CAD build for the part. Positions are in the model's coordinates, mm. Face numbers are marked on the shaded views. A direction names the side the tool comes from. Round coordinates to 2 decimals unless told otherwise and drop trailing zeros. Order: outer loops, then holes, each group sorted by start corner. A loop starts at its lowest first (then second) coordinate and runs counter-clockwise, first axis right, second up. Notation, with made-up numbers: M 43.25,16 L 65.25,16 A27 cw 65.25,42 Z; hole C 65.5,76 d4. An arc over 180 degrees is marked long. Answer as a JSON object with one key per item and string values.
```python
from build123d import *

# Parameters (mm, degrees)
CUT_EXTRUDE1_DEPTH                = 145.941445074
CIRPATTERN1_COUNT                 = 6
CUT_EXTRUDE2_DEPTH                = 145.941445074
F_1_4_20_TAPPED_HOLE1_D           = 5.1054
F_1_4_20_TAPPED_HOLE1_DEPTH       = 12.7
F_1_4_20_TAPPED_HOLE1_CSINK_D     = 7.62
F_1_4_20_TAPPED_HOLE1_CSINK_ANGLE = 90
F_1_4_20_TAPPED_HOLE1_TIP         = 1.533816902


with BuildPart() as part:
    # Sketch1 → Revolve1 (revolve)
    with BuildSketch(Plane.XY, mode=Mode.PRIVATE) as revolve1_sk:
        Polygon((-6.35, 0), (6.35, 0), (6.35, 76.2), (7.62, 88.9), (12.7, 88.9), (12.7, 101.6), (-12.7, 101.6), (-12.7, 88.9), (-7.62, 88.9), (-6.35, 76.2), align=None)
    revolve(revolve1_sk.sketch.rotate(Axis((-21.230059302, 0, 0), (1, 0, 0)), 90), axis=Axis((-21.230059302, 0, 0), (1, 0, 0)))

    # Sketch2 → Cut-Extrude1 (cut, through all)
    with BuildSketch(Plane(origin=(6.35, 0, 0), x_dir=(0, 0, -1), z_dir=(1, 0, 0))):
        with BuildLine():
            Line((5.499261314, 34.925), (19.900738686, 59.869090512))
            ThreePointArc((19.900738686, 59.869090512), (19.900738686, 66.219090512), (14.401477372, 69.394090512))
            Line((14.401477372, 69.394090512), (-14.401477372, 69.394090512))
            ThreePointArc((-14.401477372, 69.394090512), (-19.900738686, 66.219090512), (-19.900738686, 59.869090512))
            Line((-19.900738686, 59.869090512), (-5.499261314, 34.925))
            ThreePointArc((-5.499261314, 34.925), (0, 31.75), (5.499261314, 34.925))
        make_face()
    cut_extrude1 = extrude(amount=-CUT_EXTRUDE1_DEPTH, mode=Mode.SUBTRACT)

    # CirPattern1: Cut-Extrude1 ×6 about axis
    cirpattern1_axis = Axis((0, 0, 0), (1, 0, 0))
    for i in range(1, CIRPATTERN1_COUNT):
        add(cut_extrude1.rotate(cirpattern1_axis, i * 360 / CIRPATTERN1_COUNT), mode=Mode.SUBTRACT)

    # Sketch3 → Cut-Extrude2 (cut, through all)
    with BuildSketch(Plane(origin=(6.35, 0, 0), x_dir=(0, 0, -1), z_dir=(1, 0, 0))):
        with BuildLine():
            Line((-6.35, 10.998522628), (-6.35, -10.998522628))
            ThreePointArc((-6.35, -10.998522628), (0, -12.7), (6.35, -10.998522628))
            Line((6.35, -10.998522628), (6.35, 10.998522628))
            ThreePointArc((6.35, 10.998522628), (0, 12.7), (-6.35, 10.998522628))
        make_face()
    extrude(amount=-CUT_EXTRUDE2_DEPTH, mode=Mode.SUBTRACT)

    # 1/4-20 Tapped Hole1
    with Locations(Plane(origin=(12.7, 0, 0), x_dir=(0, 0, -1), z_dir=(1, 0, 0))):
        with Locations((0, 95.25)):
            CounterSinkHole(F_1_4_20_TAPPED_HOLE1_D / 2, F_1_4_20_TAPPED_HOLE1_CSINK_D / 2, depth=F_1_4_20_TAPPED_HOLE1_DEPTH, counter_sink_angle=F_1_4_20_TAPPED_HOLE1_CSINK_ANGLE)
            with Locations((0, 0, -(F_1_4_20_TAPPED_HOLE1_DEPTH + F_1_4_20_TAPPED_HOLE1_TIP / 2))):  # 118° drill point
                Cone(0, F_1_4_20_TAPPED_HOLE1_D / 2, F_1_4_20_TAPPED_HOLE1_TIP, mode=Mode.SUBTRACT)


solid = part.part
```
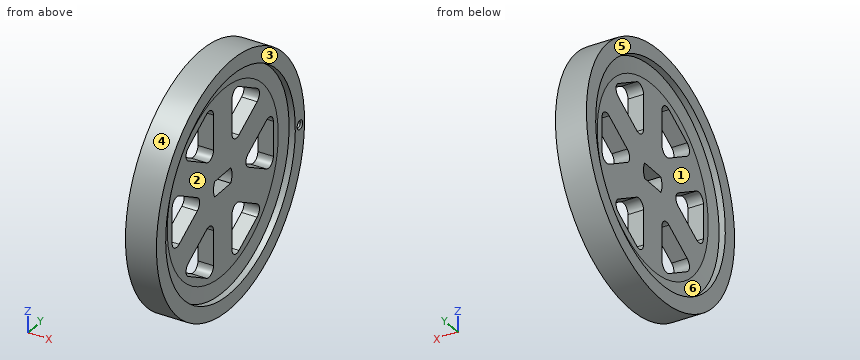
Item 1: 3-axis set-ups, long thin cutter, end or side, ignore diameter. For the marked faces 1, 2 and 3: which of +Z, -Z, +X, -X, +Y, -Y reach the whole face in a straight line?
Worked answers:
{"face 1": "-X", "face 2": "+X", "face 3": "+Z, -Z, +X, +Y, -Y"}
Item 2: Two-plate mould, pull along Z, no slides. Class the marked faces 4, 5 and 6: released by +Z, released by -Z, zero draft, split by the parting line, or undercut.
Worked answers:
{"face 4": "split by the parting line", "face 5": "zero draft", "face 6": "undercut"}
Item 3: Saw through at A-A on y = 0. List the corners of the cut face in (x, z), and give its area (3 significant figures).
Worked answers:
{"outline": "M -12.7,-101.6 L 12.7,-101.6 L 12.7,-88.9 L 7.62,-88.9 L 6.35,-76.2 L 6.35,-6.35 L -6.35,-6.35 L -6.35,-76.2 L -7.62,-88.9 L -12.7,-88.9 Z; M -12.7,88.9 L -7.62,88.9 L -6.35,76.2 L -6.35,6.35 L 6.35,6.35 L 6.35,76.2 L 7.62,88.9 L 12.7,88.9 L 12.7,101.6 L -12.7,101.6 Z", "area": "2,770 mm2"}
Item 4: Saw through at B-B on z = -48.5. State how many separate pieces and enclosed holes the cut face has, and give its area (3 significant figures).
Worked answers:
{"separate pieces": "3", "enclosed holes": "0", "area": "1,730 mm2"}
Item 5: Drop flat-ended pins along their axis: pin 1 Ø6.5 at (x, z) = (3, -42) entering from -Y; pin 2 Ø4 at (y, z) = (43, 12.5) entering from +X; pin 3 Ø14 at (x, z) = (2, 42.5) entering from -Y. Give the stop position or say it passes through.
Worked answers:
{"pin 1": "stops at y = -93.92", "pin 2": "stops at x = 6.35", "pin 3": "stops at y = -95.2"}
Item 6: Wall check: line 1 along Y through (x, z) = (9.25, 0); line 2 along Y through (x, z) = (5.75, 3); line 3 along Y through (x, z) = (3.5, 41). Give the ranges that are in metal, low to high. Write a range as [from, to].
Worked answers:
{"line 1": "y = [-101.6, -88.9], [88.9, 92.7], [97.8, 101.6]", "line 2": "y = [-101.56, -69.39], [-32.5, -12.34], [12.34, 32.5], [69.39, 101.56]", "line 3": "y = [-92.96, -45.61], [-12.7, 12.7], [45.61, 92.96]"}
